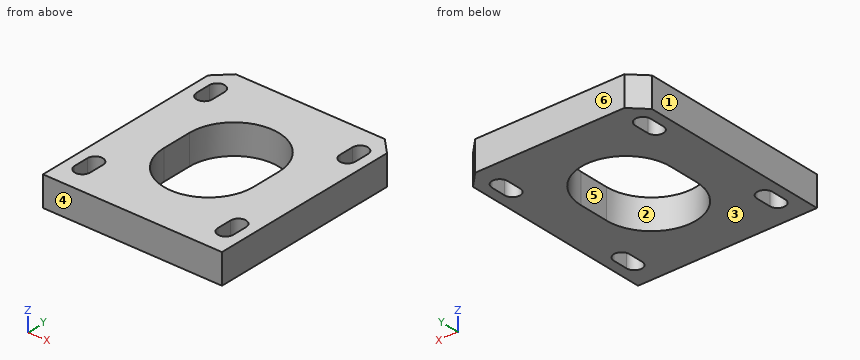
from build123d import *

# Parameters (mm, degrees)
ESQUISSE1_W             = 60
ESQUISSE1_H             = 70
BOSS_EXTRU_1_DEPTH      = 10
ENL_V_MAT_EXTRU_1_DEPTH = 10
CHANFREIN1_SIZE         = 5


with BuildPart() as part:
    # Esquisse1 → Boss.-Extru.1 (new body)
    with BuildSketch(Plane.XY):
        with Locations((30, 35)):
            Rectangle(ESQUISSE1_W, ESQUISSE1_H)
    extrude(amount=BOSS_EXTRU_1_DEPTH)

    # Esquisse2 → Enlèv. mat.-Extru.1 (cut)
    with BuildSketch(Plane.XY.offset(10)):
        with BuildLine():
            Line((8.6, 61.5), (8.6, 56.5))
            ThreePointArc((8.6, 56.5), (6, 53.9), (3.4, 56.5))
            Line((3.4, 56.5), (3.4, 61.5))
            ThreePointArc((3.4, 61.5), (6, 64.1), (8.6, 61.5))
        make_face()
        with BuildLine():
            Line((51.4, 61.5), (51.4, 56.5))
            ThreePointArc((51.4, 56.5), (54, 53.9), (56.6, 56.5))
            Line((56.6, 56.5), (56.6, 61.5))
            ThreePointArc((56.6, 61.5), (54, 64.1), (51.4, 61.5))
        make_face()
        with BuildLine():
            Line((51.4, 8.5), (51.4, 13.5))
            ThreePointArc((51.4, 13.5), (54, 16.1), (56.6, 13.5))
            Line((56.6, 13.5), (56.6, 8.5))
            ThreePointArc((56.6, 8.5), (54, 5.9), (51.4, 8.5))
        make_face()
        with BuildLine():
            Line((8.6, 8.5), (8.6, 13.5))
            ThreePointArc((8.6, 13.5), (6, 16.1), (3.4, 13.5))
            Line((3.4, 13.5), (3.4, 8.5))
            ThreePointArc((3.4, 8.5), (6, 5.9), (8.6, 8.5))
        make_face()
        with BuildLine():
            Line((15, 30), (15, 40))
            ThreePointArc((15, 40), (30, 55), (45, 40))
            Line((45, 40), (45, 30))
            ThreePointArc((45, 30), (30, 15), (15, 30))
        make_face()
    extrude(amount=-ENL_V_MAT_EXTRU_1_DEPTH, mode=Mode.SUBTRACT)

    # Chanfrein1
    chanfrein1_edges = [part.edges().sort_by_distance(p)[0] for p in [
        (0, 70, 5),
        (60, 70, 5),
    ]]
    chamfer(chanfrein1_edges, length=CHANFREIN1_SIZE)


solid = part.part
Model file for the job. Use its own axes, mm. Face numbers are marked on the shaded views. A direction names the side the tool comes from. Coordinates: 2 decimals unless noted, no trailing zeros. Order: outer loops, then holes, each group sorted by start corner. A loop starts at its lowest first (then second) coordinate and runs counter-clockwise, first axis right, second up. Notation, with made-up numbers: M -29,48.5 L 14,48.5 A12 cw 14,53.5 Z; hole C 74.25,-17.75 d11. An arc over 180 degrees is marked long. Return JSON: item names as keys, results as strings.
1. Pull direction Y, two halves, no side cores. Call the marked faces 3, 4, 5 and 6: +Y half, -Y half, draft (parallel to the pull), parting line (faces both ways), or undercut.
Ans:
{"face 3": "draft", "face 4": "-Y half", "face 5": "undercut", "face 6": "+Y half"}
2. Tool access for the marked faces 1 and 2: list every direction of +Z, -Z, +X, -X, +Y, -Y with a clear straight run to the whole face (end or side of a thin tool).
Ans:
{"face 1": "+Z, -Z, -X, +Y, -Y", "face 2": "+Z, -Z"}
3. Flat gauge pin, fed straight in: pin 1 (8 mm diameter, centred on x = 39.5, y = 34, fed in from -Z). Where does the tip first touch, or does it go through?
Ans:
{"pin 1": "through"}
4. Saw through at D-D (y = 60.5). Give the cut face in (x, z), and give its area (3 significant figures).
Ans:
{"outline": "M 0,0 L 3.4,0 L 3.4,10 L 0,10 Z; M 8.6,0 L 51.4,0 L 51.4,10 L 8.6,10 Z; M 56.6,0 L 60,0 L 60,10 L 56.6,10 Z", "area": "496 mm^2"}
5. Saw through at A-A (x = 6). Give the cut face in (y, z), and give its area (3 significant figures).
Ans:
{"outline": "M 0,0 L 5.9,0 L 5.9,10 L 0,10 Z; M 16.1,0 L 53.9,0 L 53.9,10 L 16.1,10 Z; M 64.1,0 L 70,0 L 70,10 L 64.1,10 Z", "area": "496 mm^2"}
6. Saw through at B-B (y = 38). Give the cut face in (x, z).
Ans:
{"outline": "M 0,0 L 15,0 L 15,10 L 0,10 Z; M 45,0 L 60,0 L 60,10 L 45,10 Z"}
7. Saw through at C-C (z = 2.5). Give the cut face in (x, y).
Ans:
{"outline": "M 0,0 L 60,0 L 60,65 L 55,70 L 5,70 L 0,65 Z; hole M 3.4,8.5 A2.6 ccw 8.6,8.5 L 8.6,13.5 A2.6 ccw 3.4,13.5 Z; hole M 3.4,56.5 A2.6 ccw 8.6,56.5 L 8.6,61.5 A2.6 ccw 3.4,61.5 Z; hole M 15,30 A15 ccw 45,30 L 45,40 A15 ccw 15,40 Z; hole M 51.4,8.5 A2.6 ccw 56.6,8.5 L 56.6,13.5 A2.6 ccw 51.4,13.5 Z; hole M 51.4,56.5 A2.6 ccw 56.6,56.5 L 56.6,61.5 A2.6 ccw 51.4,61.5 Z"}
8. Drill centre lines: probe 1 along X at (y, z) = (59.5, 1.75); probe 2 along Y at (x, z) = (29.5, 5); probe 3 along X at (y, z) = (63, 8.5). Where is each one in solid material? Low to high.
Ans:
{"probe 1": "0 to 3.4, 8.6 to 51.4, 56.6 to 60", "probe 2": "0 to 15.01, 54.99 to 70", "probe 3": "0 to 3.88, 8.12 to 51.88, 56.12 to 60"}
